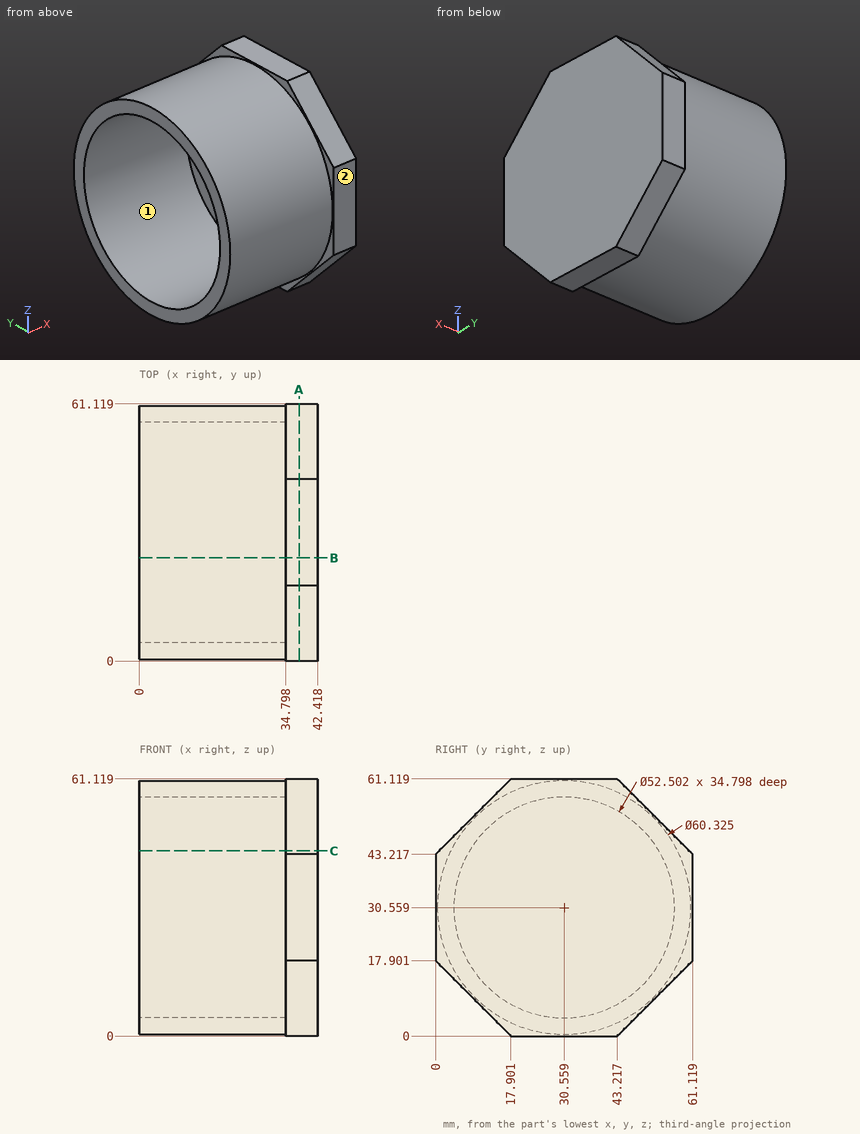
Print and shaded views of the part. All mm, measured from the part's lowest x, y and z. A direction names the side the tool comes from. Coordinates: 2 decimals unless noted, no trailing zeros. Order: outer loops, then holes, each group sorted by start corner. A loop starts at its lowest first (then second) coordinate and runs counter-clockwise, first axis right, second up.
(1) Slice it at A-A, the plane x = 38. Write the cut outline in (y, z), and give its area (3 significant figures).
Check sheet entries:
outline: (0, 17.9) - (17.9, 0) - (43.22, 0) - (61.12, 17.9) - (61.12, 43.22) - (43.22, 61.12) - (17.9, 61.12) - (0, 43.22) - close
area: 3,090 mm2
(2) Pin check, flat tips, straight feed: pin 1 Ø1 at (x, y) = (11.5, 35) entering from -Z (1 decimal); pin 2 Ø2 at (x, z) = (30.5, 19) entering from +Y; pin 3 Ø18.5 at (y, z) = (37.5, 43) entering from -X. Stop position of each tip, or through.
Check sheet entries:
pin 1: stops at z = 0.7
pin 2: stops at y = 58.81
pin 3: stops at x = 34.8
(3) Slice it at B-B, the plane y = 24.5. Write the cut outline in (x, z).
Check sheet entries:
outline: (0, 1.01) - (34.8, 1.01) - (34.8, 0) - (42.42, 0) - (42.42, 61.12) - (34.8, 61.12) - (34.8, 60.11) - (0, 60.11) - (0, 56.1) - (34.8, 56.1) - (34.8, 5.02) - (0, 5.02) - close
(4) Tool access for the marked faces 1 and 2: list every direction of +Z, -Z, +X, -X, +Y, -Y with a clear straight run to the whole face (end or side of a thin tool).
Check sheet entries:
face 1: -X
face 2: +Z, -Z, +X, -X, -Y
(5) Slice it at C-C, the plane z = 44. Write the cut outline in (x, y).
Check sheet entries:
outline: (0, 3.56) - (34.8, 3.56) - (34.8, 0.78) - (42.42, 0.78) - (42.42, 60.34) - (34.8, 60.34) - (34.8, 57.56) - (0, 57.56) - (0, 53.11) - (34.8, 53.11) - (34.8, 8.01) - (0, 8.01) - close
(6) Probe L1, parallel to X at y = 47, z = 10.5; L2, parallel to Z at x = 19.5, y = 12 (1 decimal); L3, parallel to Y at x = 12.5, z = 48.5 (1 decimal). List the from-to ranges inside material, lowest first.
Check sheet entries:
L1: x = 34.8 to 42.42
L2: z = 6.8 to 12, 49.1 to 54.3
L3: y = 6.3 to 11.4, 49.7 to 54.8
